Geometry check sheet. Reference: the model listing, model coordinates, mm. Round coordinates to 2 decimals unless told otherwise and drop trailing zeros. Order: outer loops, then holes, each group sorted by start corner. A loop starts at its lowest first (then second) coordinate and runs counter-clockwise, first axis right, second up. Notation, with made-up numbers: (10, 11) -> (53, 11) arc R12 ccw to (53, 19) -> close; hole circle Ø4 at (-9, 23.5). An arc over 180 degrees is marked (long way). Use a Markdown table: item, result. Add a question column.
Item 1: Material ranges on probe 1 along X at (y, z) = (-0.9, -8); probe 2 along X at (y, z) = (-1.7, 6); probe 3 along Z at (x, y) = (-18.5, -0.55), recorded low to high. Write a range as [from, to].
Item 2: Sectioned sample at A-A, the plane x = 16.95. Record the cut outline in (y, z).
Item 3: Sectioned sample at B-B, the plane y = -2. Record the cut outline in (x, z), and give its area (3 significant figures).
Item 4: Mould release check, pull along X, two halves, no side actions. Record for faces 1 (the flat face through (-3, -3, 2)), 2 (the cylindrical face through (18.685, -1.479, 6.814)), 3 (the flat face through (-25, -1, 3)): pulls with the +X half, pulls with the -X half, needs draft (parallel to the pull), parting line crosses it, or undercut.
Item 5: Sectioned sample at C-C, the plane z = -12.5. Record the cut outline in (x, y), and give its area (3 significant figures).
from build123d import *

# Parameters (mm, degrees)
SKETCH2_W           = 45
SKETCH2_H           = 50
SKETCH2_R           = 7.5
BOSS_EXTRUDE1_DEPTH = 3
SKETCH1_R           = 1.75
CUT_EXTRUDE1_DEPTH  = 3


with BuildPart() as part:
    # Sketch2 → Boss-Extrude1 (new body)
    with BuildSketch(Plane(origin=(0, 0, 0), x_dir=(1, 0, 0), z_dir=(0, 1, 0))):
        with Locations((-2.5, -2.5)):
            Rectangle(SKETCH2_W, SKETCH2_H)
        with Locations(Location((0, 8, 0), (0, 0, 270))):
            Circle(SKETCH2_R, mode=Mode.SUBTRACT)
    extrude(amount=-BOSS_EXTRUDE1_DEPTH)

    # Sketch1 → Cut-Extrude1 (cut)
    with BuildSketch(Plane(origin=(0, 0, 0), x_dir=(1, 0, 0), z_dir=(0, 1, 0))):
        with Locations(Location((-18.45, -1.75, 0), (0, 0, 270))):
            Circle(SKETCH1_R)
        with Locations(Location((16.95, -7.041502622, 0), (0, 0, 270))):
            Circle(SKETCH1_R)
        with Locations(Location((-16.95, -7.041502622, 0), (0, 0, 270))):
            Circle(SKETCH1_R)
    extrude(amount=-CUT_EXTRUDE1_DEPTH, mode=Mode.SUBTRACT)


solid = part.part
Found:
| question | item | result |
|---|---|---|
| 1 | probe 1 | x = [-25, -7.5], [7.5, 20] |
| 1 | probe 2 | x = [-25, -18.36], [-15.54, 15.54], [18.36, 20] |
| 1 | probe 3 | z = [-22.5, 0], [3.5, 6.23], [7.85, 27.5] |
| 2 | outline | (-3, -22.5) -> (0, -22.5) -> (0, 5.29) -> (-3, 5.29) -> close; (-3, 8.79) -> (0, 8.79) -> (0, 27.5) -> (-3, 27.5) -> close |
| 3 | outline | (-25, -22.5) -> (20, -22.5) -> (20, 27.5) -> (-25, 27.5) -> close; hole circle Ø3.5 at (-18.45, 1.75); hole circle Ø3.5 at (-16.95, 7.04); hole circle Ø15 at (0, -8); hole circle Ø3.5 at (16.95, 7.04) |
| 3 | area | 2,040 mm2 |
| 4 | face 1 | needs draft |
| 4 | face 2 | undercut |
| 4 | face 3 | pulls with the -X half |
| 5 | outline | (-25, -3) -> (-6, -3) -> (-6, 0) -> (-25, 0) -> close; (6, -3) -> (20, -3) -> (20, 0) -> (6, 0) -> close |
| 5 | area | 99.0 mm2 |
